from build123d import *


with BuildPart() as part:
    # Esquisse1 → Révolution1 (revolve)
    with BuildSketch(Plane(origin=(0, 0, 0), x_dir=(0, 0, -1), z_dir=(1, 0, 0))):
        with BuildLine():
            Line((0, 0), (0, 0.8))
            ThreePointArc((0, 0.8), (-0.058578644, 0.941421356), (-0.2, 1))
            Line((-0.2, 1), (-9, 1))
            Line((-9, 1), (-9, 0.65))
            Line((-9, 0.65), (-9.4, 0.65))
            Line((-9.4, 0.65), (-9.4, 1))
            Line((-9.4, 1), (-22.1, 1))
            Line((-22.1, 1), (-22.1, 0.65))
            Line((-22.1, 0.65), (-22.5, 0.65))
            Line((-22.5, 0.65), (-22.5, 1))
            Line((-22.5, 1), (-23.3, 1))
            ThreePointArc((-23.3, 1), (-23.441421356, 0.941421356), (-23.5, 0.8))
            Line((-23.5, 0.8), (-23.5, 0))
            Line((-23.5, 0), (0, 0))
        make_face()
    revolve(axis=Axis((0, 0, 23.5), (0, 0, -1)))


solid = part.part
For this review, take the finished solid that the model builds, in its own axes (mm). Give positions to 0.01 mm unless a question says otherwise; leave off trailing zeros. Loops run counter-clockwise (first coordinate to the right, second up) from the corner with the lowest first, then second, coordinate; pieces in that order, holes last. Notation, with made-up numbers: (-30.75, 27) - (2.25, 27) arc R21 cw to (2.25, 64) - close; hole circle Ø1 at (28, -37). An arc over 180 degrees is marked (long way). Write each question's results on one line, items separated by ' | '.
(1) Take a section at A-A (z = 1.75). Give the boundary of the cut face in (x, y).
Conclusion:
outline: circle Ø2 at (0, 0)
(2) Draft analysis for pull direction Z (two halves, no side actions). For faces 1 (the cylindrical face through (0.644, -0.085, 9.203)), 2 (the cylindrical face through (-1, 0, 23)), 3 (the cylindrical face through (0.644, -0.085, 22.303)), 4 (the flat face through (0, 0, 0)), state which applies: +Z half, -Z half, draft (parallel to the pull), parting line (faces both ways), or undercut.
Conclusion:
face 1: undercut | face 2: draft | face 3: undercut | face 4: -Z half
(3) For line 1 along Z through (x, y) = (-0.45, -0.55); line 2 along Y through (x, z) = (0.6, 12.5); line 3 along X through (y, z) = (-0.05, 15.5), list the stretches that pass through material, from the lowest coordinate up.
Conclusion:
line 1: 0 to 9, 9.4 to 22.1, 22.5 to 23.5 | line 2: -0.8 to 0.8 | line 3: -1 to 1
